```python
from build123d import *

# Parameters (mm, degrees)
BOSS_EXTRU_3_DEPTH      = 5
ESQUISSE7_R             = 3.175
BOSS_EXTRU_5_DEPTH      = 10
ESQUISSE13_R            = 2.18
BOSS_EXTRU_8_DEPTH      = 5
ESQUISSE33_W            = 9.466792894
ESQUISSE33_H            = 55.28
BOSS_EXTRU_10_DEPTH     = 10
ENL_V_MAT_EXTRU_6_DEPTH = 65
ESQUISSE35_R            = 30
BOSS_EXTRU_11_DEPTH     = 5.32
BOSS_EXTRU_12_DEPTH     = 30
ESQUISSE41_R            = 3.175
ENL_V_MAT_EXTRU_7_DEPTH = 60
ESQUISSE42_R            = 1.75
BOSS_EXTRU_13_DEPTH     = 5
NERVURE4_REACH          = 90.538
ESQUISSE45_WALL_W       = 193.218913386
ESQUISSE45_WALL_H       = 3
CONG_1_R                = 1
CONG_2_R                = 1


with BuildPart() as part:
    # Esquisse5 → Boss.-Extru.3 (new, symmetric)
    with BuildSketch(Plane(origin=(0, 0, 0), x_dir=(1, 0, 0), z_dir=(0, 1, 0))):
        with BuildLine():
            Line((42.5, -30), (-42.5, -30))
            ThreePointArc((-42.5, -30), (-72.5, 0), (-42.5, 30))
            Line((-42.5, 30), (42.5, 30))
            ThreePointArc((42.5, 30), (72.5, 0), (42.5, -30))
        make_face()
    extrude(amount=BOSS_EXTRU_3_DEPTH, both=True)

    # Esquisse7 → Boss.-Extru.5 (add, symmetric)
    with BuildSketch(Plane.XY):
        with BuildLine():
            Line((32.5, 5), (52.5, 5))
            Line((52.5, 5), (52.5, 20))
            ThreePointArc((52.5, 20), (42.5, 30), (32.5, 20))
            Line((32.5, 20), (32.5, 5))
        make_face()
        with Locations((42.5, 20)):
            Circle(ESQUISSE7_R, mode=Mode.SUBTRACT)
    extrude(amount=BOSS_EXTRU_5_DEPTH, both=True)

    # Esquisse13 → Boss.-Extru.8 (add)
    with BuildSketch(Plane.XY.offset(22.64)):
        Polygon((0.8, 5), (5.8, 5), (12.215, 5), (12.215, 29.91), (52.215, 29.91), (52.215, 5), (58.63, 5), (63.63, 5), (63.63, 34.91), (0.8, 34.91), align=None)
        with Locations((8.47, 14.92)):
            Circle(ESQUISSE13_R, mode=Mode.SUBTRACT)
        with Locations((55.97, 14.92)):
            Circle(ESQUISSE13_R, mode=Mode.SUBTRACT)
        with Locations((8.47, 25.08)):
            Circle(ESQUISSE13_R, mode=Mode.SUBTRACT)
        with Locations((55.97, 25.08)):
            Circle(ESQUISSE13_R, mode=Mode.SUBTRACT)
    boss_extru_8 = extrude(amount=BOSS_EXTRU_8_DEPTH)

    # Symétrie2: Boss.-Extru.8 across plane
    add(boss_extru_8.mirror(Plane.XY))

    # Esquisse33 → Boss.-Extru.10 (add)
    with BuildSketch(Plane.XZ.offset(-5)):
        with Locations((58.896603553, 0)):
            Rectangle(ESQUISSE33_W, ESQUISSE33_H)
    extrude(amount=BOSS_EXTRU_10_DEPTH)

    # Esquisse36 → Enlèv. mat.-Extru.6 (cut, symmetric)
    with BuildSketch(Plane.XY):
        Polygon((0, 0), (9.099255857, -25), (-112.5, -25), (-112.5, 35), (-12.738958199, 35), align=None)
    extrude(amount=ENL_V_MAT_EXTRU_6_DEPTH, both=True, mode=Mode.SUBTRACT)



with BuildPart() as body_2:
    # Esquisse35 → Boss.-Extru.11 (new, symmetric)
    with BuildSketch(Plane(origin=(0, 0, 0), x_dir=(0, 0, -1), z_dir=(-0.34202014332566977, 0.939692620785908, 0))):
        with Locations(Location((0, 30, 0), (0, 0, 90))):
            Circle(ESQUISSE35_R)
    extrude(amount=BOSS_EXTRU_11_DEPTH, both=True)


with BuildPart() as part_1:
    add(part.part)

    add(body_2.part)  # Boss.-Extru.12 merges body 2
    # Esquisse40 → Boss.-Extru.12 (add, symmetric)
    with BuildSketch(Plane.XY):
        Polygon((-26.371231461, -15.259769042), (-30.010325786, -5.261439557), (-1.819547162, 4.999164743), (1.819547162, -4.999164743), align=None)
    extrude(amount=BOSS_EXTRU_12_DEPTH, both=True)

    # Esquisse41 → Enlèv. mat.-Extru.7 (cut)
    with BuildSketch(Plane(origin=(-1.819547162, 4.999164743, 0), x_dir=(0.939692620785908, 0.3420201433256698, 0), z_dir=(-0.3420201433256698, 0.9396926207859081, 0))):
        with Locations(Location((-30, 0, 0), (0, 0, 180))):
            Circle(ESQUISSE41_R)
    extrude(amount=-ENL_V_MAT_EXTRU_7_DEPTH, mode=Mode.SUBTRACT)

    # Esquisse42 → Boss.-Extru.13 (add)
    with BuildSketch(Plane.XY.offset(27.64)):
        with BuildLine():
            Line((0.8, 39.91), (0.8, 34.91))
            Line((0.8, 34.91), (12.215, 34.91))
            Line((12.215, 34.91), (12.215, 39.91))
            ThreePointArc((12.215, 39.91), (6.5075, 45.6175), (0.8, 39.91))
        make_face()
        with Locations((6.5075, 39.91)):
            Circle(ESQUISSE42_R, mode=Mode.SUBTRACT)
    extrude(amount=-BOSS_EXTRU_13_DEPTH)

    # Esquisse45 wall → Nervure4 (add, up to next)
    with BuildSketch(Plane(origin=(2.8, 9.999582371, 17.640000004), x_dir=(0, -0.707106781505, -0.707106780868), z_dir=(0, -0.707106780868, 0.707106781505)), mode=Mode.PRIVATE) as nervure4_sk1:
        Rectangle(ESQUISSE45_WALL_W, ESQUISSE45_WALL_H)
    nervure4_tool1 = extrude(nervure4_sk1.sketch, amount=NERVURE4_REACH, mode=Mode.PRIVATE) - part_1.part
    nervure4 = nervure4_tool1.solids().sort_by_distance((2.8, 9.999582371, 17.640000004))[0]
    add(nervure4)

    # Congé1
    cong_1_edges = [part_1.edges().sort_by_distance(p)[0] for p in [
        (54.163207106, 0, 27.64),
        (63.63, 14.955, 27.64),
        (63.63, 0, 21.296081799),
        (63.63, 0, -21.296081799),
        (63.63, 14.955, -27.64),
        (54.163207106, 0, -27.64),
    ]]
    fillet(cong_1_edges, radius=CONG_1_R)

    # Symétrie3: Nervure4 across plane
    add(nervure4.mirror(Plane.XY))

    # Congé2
    cong_2_edges = [part_1.edges().sort_by_distance(p)[0] for p in [
        (63.63, 34.91, 24.64),
        (63.63, 34.91, -24.64),
        (52.215, 5, 25.14),
        (12.215, 5, -25.14),
        (12.215, 29.91, 25.14),
        (52.215, 29.91, 25.14),
        (0.8, 22.455, 27.64),
        (12.215, 5, 25.14),
        (52.215, 29.91, -25.14),
        (12.215, 29.91, -25.14),
        (0.8, 34.91, -25.14),
        (52.215, 5, -25.14),
        (31.715, 34.91, -27.64),
        (37.4225, 34.91, 27.64),
        (6.5075, 45.6175, 27.64),
        (12.215, 34.91, 25.14),
        (12.215, 37.41, 27.64),
        (63.337106781, 34.91, 27.347106781),
        (63.337106781, 34.91, -27.347106781),
    ]]
    fillet(cong_2_edges, radius=CONG_2_R)


solid = part_1.part
```
Source: CAD feature listing. Evaluate the final solid. Frame: model axes, mm. A direction names the side the tool comes from. Give positions to 0.01 mm unless a question says otherwise; leave off trailing zeros. Loops run counter-clockwise (first coordinate to the right, second up) from the corner with the lowest first, then second, coordinate; pieces in that order, holes last. Notation, with made-up numbers: (86, 18.25) - (133, 18.25) arc R20 cw to (133, 56.25) - close; hole circle Ø6 at (2, -11). An arc over 180 degrees is marked (long way). Use CSV: the item, a comma, the result in double quotes. Start each with the question number.
1. Draft query along Y for faces 1 (the cylindrical face through (10.484, 14.085, -25.105)), 2 (the flat face through (2.82, 10.07, -17.71)), 3 (the flat face through (12.215, 17, 25)), 4 (the flat face through (52.5, 12, 0)). Return one class per face: +Y half, -Y half, draft (parallel to the pull), parting line (faces both ways), or undercut.
2. Reachability of faces 5 (the flat face through (1.3, 8, 20)), 6 (the flat face through (2.82, 10.07, 17.71)), 7 (the flat face through (63.63, 15, -25)) from +Z, -Z, +X, -X, +Y, -Y: full face, straight path, thin tool, end or side. Return the list, or none.
3. Pin query (flat end, axial travel): pin 1 (1.5 mm diameter, centred on x = 49, y = 13.5, fed in from -Z); pin 2 (3 mm diameter, centred on y = 28, z = 25, fed in from -X); pin 3 (1.5 mm diameter, centred on y = 19.5, z = -24.5, fed in from +X). Return the tip coordinate at first contact, or that it passes through.
4. Ray query, L1, parallel to Y at x = 55.97, z = -25.85; L2, parallel to Y at x = 8, z = -25; L3, parallel to Z at x = 58.5, y = 7.5. Return the intervals inside material, ascending.
5. Section C-C (y = 3). Output: boundary loops of the cut face in (x, z).
6. Section A-A (x = 55.97). Output: boundary loops of the cut face in (y, z).
Response:
1,face 1,"undercut"
1,face 2,"+Y half"
1,face 3,"undercut"
1,face 4,"draft"
2,face 5,"-X, +Y"
2,face 6,"+X, -X, +Y"
2,face 7,"-Z, +X, +Y, -Y"
3,pin 1,"z = -10"
3,pin 2,"x = 0.8"
3,pin 3,"x = 63.63"
4,L1,"-5 to 12.74, 17.1 to 22.9, 27.26 to 34.91"
4,L2,"-5 to 12.79, 17.05 to 22.95, 27.21 to 34.91"
4,L3,"-27.64 to -22.64, 22.64 to 27.64"
5,outline,"(-7.31, -30) - (42.5, -30) arc R30 ccw to (53.98, -27.72) arc R1 cw to (54.36, -27.64) - (62.63, -27.64) arc R1 ccw to (63.63, -26.64) - (63.63, -21.71) arc R1 cw to (63.92, -21.01) arc R30 ccw to (63.92, 21.01) arc R1 cw to (63.63, 21.71) - (63.63, 26.64) arc R1 ccw to (62.63, 27.64) - (54.36, 27.64) arc R1 cw to (53.98, 27.72) arc R30 ccw to (42.5, 30) - (-7.31, 30) - close"
6,outline,"(-5, -27.64) - (12.74, -27.64) - (12.74, -22.64) - (5, -22.64) - (5, 22.64) - (12.74, 22.64) - (12.74, 27.64) - (-5, 27.64) - close; (17.1, -27.64) - (22.9, -27.64) - (22.9, -22.64) - (17.1, -22.64) - close; (17.1, 22.64) - (22.9, 22.64) - (22.9, 27.64) - (17.1, 27.64) - close; (27.26, -27.64) - (33.91, -27.64) arc R1 ccw to (34.91, -26.64) - (34.91, -22.64) - (27.26, -22.64) - close; (27.26, 22.64) - (34.91, 22.64) - (34.91, 26.64) arc R1 ccw to (33.91, 27.64) - (27.26, 27.64) - close"
